from build123d import *

# Parameters (mm, degrees)
SKETCH_1_R          = 24.5
SKETCH_1_R_2        = 2.1
EXTRUDE_1_DEPTH     = 2
CUT_EXTRUDE_1_DEPTH = 10


with BuildPart() as part:
    # 草图1 → 凸台-拉伸1 (new body)
    with BuildSketch(Plane.XY):
        with BuildLine():
            Line((-60, 15), (-60, -15))
            ThreePointArc((-60, -15), (-58.975297052, -18.032657803), (-56.321194659, -19.82228625))
            Line((-56.321194659, -19.82228625), (-8.984123683, -32.791546497))
            ThreePointArc((-8.984123683, -32.791546497), (0, -34), (8.984123683, -32.791546497))
            Line((8.984123683, -32.791546497), (56.321194659, -19.82228625))
            ThreePointArc((56.321194659, -19.82228625), (58.975297052, -18.032657803), (60, -15))
            Line((60, -15), (60, 15))
            ThreePointArc((60, 15), (58.975297052, 18.032657803), (56.321194659, 19.82228625))
            Line((56.321194659, 19.82228625), (8.984123683, 32.791546497))
            ThreePointArc((8.984123683, 32.791546497), (0, 34), (-8.984123683, 32.791546497))
            Line((-8.984123683, 32.791546497), (-56.321194659, 19.82228625))
            ThreePointArc((-56.321194659, 19.82228625), (-58.975297052, 18.032657803), (-60, 15))
        make_face()
        Circle(SKETCH_1_R, mode=Mode.SUBTRACT)
        with Locations((0, 29)):
            Circle(SKETCH_1_R_2, mode=Mode.SUBTRACT)
        with Locations((25.11473671, 14.5)):
            Circle(SKETCH_1_R_2, mode=Mode.SUBTRACT)
        with Locations((25.11473671, -14.5)):
            Circle(SKETCH_1_R_2, mode=Mode.SUBTRACT)
        with Locations((0, -29)):
            Circle(SKETCH_1_R_2, mode=Mode.SUBTRACT)
        with Locations((-25.11473671, -14.5)):
            Circle(SKETCH_1_R_2, mode=Mode.SUBTRACT)
        with Locations((-25.11473671, 14.5)):
            Circle(SKETCH_1_R_2, mode=Mode.SUBTRACT)
        with Locations((-55, 15)):
            Circle(SKETCH_1_R_2, mode=Mode.SUBTRACT)
        with Locations((-55, -15)):
            Circle(SKETCH_1_R_2, mode=Mode.SUBTRACT)
        with Locations((55, -15)):
            Circle(SKETCH_1_R_2, mode=Mode.SUBTRACT)
        with Locations((55, 15)):
            Circle(SKETCH_1_R_2, mode=Mode.SUBTRACT)
    extrude(amount=EXTRUDE_1_DEPTH)

    # 草图2 → 切除-拉伸1 (cut)
    with BuildSketch(Plane.XY.offset(2)):
        with BuildLine():
            Line((-48, 11), (-36, 11))
            ThreePointArc((-36, 11), (-34.585786438, 10.414213562), (-34, 9))
            Line((-34, 9), (-34, -9))
            ThreePointArc((-34, -9), (-34.585786438, -10.414213562), (-36, -11))
            Line((-36, -11), (-48, -11))
            ThreePointArc((-48, -11), (-49.414213562, -10.414213562), (-50, -9))
            Line((-50, -9), (-50, 9))
            ThreePointArc((-50, 9), (-49.414213562, 10.414213562), (-48, 11))
        make_face()
        with BuildLine():
            Line((36, 11), (48, 11))
            ThreePointArc((48, 11), (49.414213562, 10.414213562), (50, 9))
            Line((50, 9), (50, -9))
            ThreePointArc((50, -9), (49.414213562, -10.414213562), (48, -11))
            Line((48, -11), (36, -11))
            ThreePointArc((36, -11), (34.585786438, -10.414213562), (34, -9))
            Line((34, -9), (34, 9))
            ThreePointArc((34, 9), (34.585786438, 10.414213562), (36, 11))
        make_face()
    extrude(amount=-CUT_EXTRUDE_1_DEPTH, mode=Mode.SUBTRACT)


solid = part.part
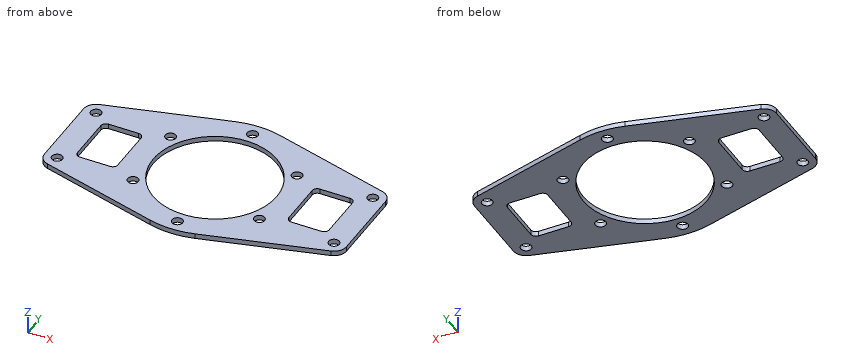
The model under review builds one solid part; all positions refer to its coordinate system, in mm. Round coordinates to 2 decimals unless told otherwise and drop trailing zeros. Write each loop counter-clockwise with the first axis right and the second up, starting at its lowest first coordinate (ties: lowest second). Pieces come first, ordered by that corner, then holes. Notation, with made-up numbers: (49.25, -11) - (64.25, -11) arc R22 ccw to (64.25, 15) - close; hole circle Ø3 at (43.5, 66.25). An arc over 180 degrees is marked (long way). One line per item, written item: value. Start each with the question number.
1. Clearance check with flat-ended pins moving along their axes: P1, Ø1.5, axis at x = 47.5, y = -1, coming from the +Z side; P2, Ø0.6, axis at x = 41, z = 0.5, coming from the -Y side; P3, Ø5, axis at x = 25.11, y = 14.5, coming from the -Z side; P4, Ø1, axis at x = -44, z = 1, coming from the +Y side (3 decimals). State where each tip first meets the part, or that it passes through.
2. Consider section A-A on y = 0. Write out the cut boundary in (x, z).
3. Consider section D-D on z = 1.1. State how many separate pieces and enclosed holes the cut face has, and give its area (3 significant figures).
4. Consider section B-B on x = 0. Write out the cut boundary in (y, z).
5. Consider section C-C on x = -42. Write out the cut boundary in (y, z), and give its area (3 significant figures).
6. To check wall thickness, follow L1, parallel to X at y = -9.5, z = 1.6; L2, parallel to Y at x = 55, z = 0.65; L3, parallel to X at y = 9, z = 0.25. State the ranges of each line that lie inside material, in increasing order. Write a range as from..to.
Checks:
1. P1: passes through
1. P2: stops at y = -24.1
1. P3: stops at z = 0
1. P4: stops at y = 23.335
2. outline: (-60, 0) - (-50, 0) - (-50, 2) - (-60, 2) - close; (-34, 0) - (-24.5, 0) - (-24.5, 2) - (-34, 2) - close; (24.5, 0) - (34, 0) - (34, 2) - (24.5, 2) - close; (50, 0) - (60, 0) - (60, 2) - (50, 2) - close
3. separate pieces: 1
3. enclosed holes: 13
3. area: 3,740 mm^2
4. outline: (-34, 0) - (-31.1, 0) - (-31.1, 2) - (-34, 2) - close; (-26.9, 0) - (-24.5, 0) - (-24.5, 2) - (-26.9, 2) - close; (24.5, 0) - (26.9, 0) - (26.9, 2) - (24.5, 2) - close; (31.1, 0) - (34, 0) - (34, 2) - (31.1, 2) - close
5. outline: (-23.75, 0) - (-11, 0) - (-11, 2) - (-23.75, 2) - close; (11, 0) - (23.75, 0) - (23.75, 2) - (11, 2) - close
5. area: 51.0 mm^2
6. L1: x = -60..-49.94, -34.06..-22.58, 22.58..34.06, 49.94..60
6. L2: y = -20.18..-17.1, -12.9..12.9, 17.1..20.18
6. L3: x = -60..-50, -34..-22.79, 22.79..34, 50..60
